```python
from build123d import *

# Parameters (mm, degrees)
BOSS_EXTRUDE1_DEPTH = 50.8
SKETCH5_W           = 50.8
SKETCH5_H           = 34.441508913
SKETCH8_W           = 12.7
SKETCH8_H           = 25.4
SKETCH11_W          = 50.8
SKETCH11_H          = 34.441508913
SKETCH10_W          = 12.7
SKETCH10_H          = 25.4
SKETCH12_W          = 34.441508912
SKETCH12_H          = 50.8
SKETCH13_W          = 25.4
SKETCH13_H          = 12.7
SKETCH14_W          = 34.441508912
SKETCH14_H          = 50.8
SKETCH15_W          = 25.4
SKETCH15_H          = 12.7


with BuildPart() as part:
    # Sketch3 → Boss-Extrude1 (new body)
    with BuildSketch(Plane.XY):
        Polygon((-583.133216143, 41.413481842), (-617.573251094, 41.732117626), (-642.151342876, 17.604644891), (-642.469978659, -16.83539006), (-618.342505925, -41.413481842), (-583.902470973, -41.732117626), (-559.324379192, -17.604644891), (-559.005743408, 16.83539006), align=None)
    extrude(amount=BOSS_EXTRUDE1_DEPTH)

    # Sketch5 → Loft1 section 0
    with BuildSketch(Plane(origin=(-335.594803105, -329.44194911, 0), x_dir=(0, 0, 1), z_dir=(-0.713618322, -0.700534718, 0))):
        with Locations((25.4, 420.837728092)):
            Rectangle(SKETCH5_W, SKETCH5_H)
    # Sketch8 → Loft1 section 1
    with BuildSketch(Plane(origin=(-656.72304774, -644.682572171, 0), x_dir=(0, 0, 1), z_dir=(-0.713618322, -0.700534718, 0))):
        with Locations((6.35, 420.201309854)):
            Rectangle(SKETCH8_W, SKETCH8_H)
    loft()

    # Sketch11 → Loft2 section 0
    with BuildSketch(Plane(origin=(-276.258040589, -271.193077208, 0), x_dir=(0, 0, -1), z_dir=(0.713618322, 0.700534718, 0))):
        with Locations((-25.4, 420.837728092)):
            Rectangle(SKETCH11_W, SKETCH11_H)
    # Sketch10 → Loft2 section 1
    with BuildSketch(Plane(origin=(44.870204046, 44.047545853, 0), x_dir=(0, 0, -1), z_dir=(0.713618322, 0.700534718, 0))):
        with Locations((-6.35, 420.201309854)):
            Rectangle(SKETCH10_W, SKETCH10_H)
    loft()

    # Sketch12 → Loft3 section 0
    with BuildSketch(Plane(origin=(-265.687003236, 270.649131901, 0), x_dir=(-0.713618322, -0.700534718, 0), z_dir=(0.700534718, -0.713618322, 0))):
        with Locations((428.697544073, -25.4)):
            Rectangle(SKETCH12_W, SKETCH12_H)
    # Sketch13 → Loft3 section 1
    with BuildSketch(Plane(origin=(49.553619825, -50.479112734, 0), x_dir=(-0.713618322, -0.700534718, 0), z_dir=(0.700534718, -0.713618322, 0))):
        with Locations((428.656835586, -6.35)):
            Rectangle(SKETCH13_W, SKETCH13_H)
    loft()

    # Sketch14 → Loft4 section 0
    with BuildSketch(Plane(origin=(-323.935875138, 329.985894417, 0), x_dir=(0.713618322, 0.700534718, 0), z_dir=(-0.700534718, 0.713618322, 0))):
        with Locations((-428.697544073, -25.4)):
            Rectangle(SKETCH14_W, SKETCH14_H)
    # Sketch15 → Loft4 section 1
    with BuildSketch(Plane(origin=(-639.176498199, 651.114139052, 0), x_dir=(0.713618322, 0.700534718, 0), z_dir=(-0.700534718, 0.713618322, 0))):
        with Locations((-428.656835586, -6.35)):
            Rectangle(SKETCH15_W, SKETCH15_H)
    loft()


solid = part.part
```
Input: part model. Units: mm. Frame: model coordinates. Round coordinates to 2 decimals unless told otherwise and drop trailing zeros. Loops run counter-clockwise (first coordinate to the right, second up) from the corner with the lowest first, then second, coordinate; pieces in that order, holes last. Notation, with made-up numbers: M 78.5,-37.75 L 85.5,-37.75 A12 cw 85.5,-33.75 Z; hole C 63.25,27 d8. An arc over 180 degrees is marked long. Answer in a Markdown table with one row per item. Add a question column.
1. Ray query, probe 1 along X at (y, z) = (58, 35) (3 decimals); probe 2 along X at (y, z) = (-62.5, 18); probe 3 along Y at (x, z) = (-432, 15). Return the intervals inside material, ascending.
2. Section A-A (x = -605.5). Output: boundary loops of the cut face in (y, z), and give its area (3 significant figures).
3. Contact query for flat-ended pins moving along their axis: pin 1 (1 mm diameter, centred on y = -144.5, z = 34, fed in from +X); pin 2 (1 mm diameter, centred on x = -424, z = 32, fed in from -Y); pin 3 (3 mm diameter, centred on y = 49, z = 42, fed in from -X). Output: stop coordinate, or through.
Values follow:
| question | item | result |
|---|---|---|
| 1 | probe 1 | -681.01 to -633.864, -565.845 to -517.79 |
| 1 | probe 2 | -687.93 to -640.2, -563.1 to -516.12 |
| 1 | probe 3 | -193.37 to -149.92, 143.68 to 186.41 |
| 2 | outline | M -41.53,0 L 41.62,0 L 41.62,50.8 L -41.53,50.8 Z |
| 2 | area | 4,220 mm^2 |
| 3 | pin 1 | x = -436.73 |
| 3 | pin 2 | y = -201.69 |
| 3 | pin 3 | x = -673.8 |
